from build123d import *

# Parameters (mm, degrees)
BOSS_EXTRUDE1_DEPTH = 19
SKETCH2_R           = 1.905
CUT_EXTRUDE1_DEPTH  = 10.16
CHAMFER1_SIZE       = 1.016
CHAMFER2_SIZE       = 0.254
CHAMFER3_SIZE       = 1.016


with BuildPart() as part:
    # Sketch1 → Boss-Extrude1 (new body)
    with BuildSketch(Plane(origin=(0, 0, 0), x_dir=(0, 0, -1), z_dir=(1, 0, 0))):
        with BuildLine():
            Line((6.25, -13.87), (-25.5, -13.87))
            Line((-25.5, -13.87), (-25.5, 38))
            Line((-25.5, 38), (25.5, 38))
            Line((25.5, 38), (25.5, 24.08))
            Line((25.5, 24.08), (-6.25, 24.08))
            ThreePointArc((-6.25, 24.08), (-11.33, 19), (-6.25, 13.92))
            Line((-6.25, 13.92), (25.5, 13.92))
            Line((25.5, 13.92), (25.5, -38))
            Line((25.5, -38), (-25.5, -38))
            Line((-25.5, -38), (-25.5, -24.03))
            Line((-25.5, -24.03), (6.25, -24.03))
            ThreePointArc((6.25, -24.03), (11.33, -18.95), (6.25, -13.87))
        make_face()
    extrude(amount=BOSS_EXTRUDE1_DEPTH)

    # Sketch2 → Cut-Extrude1 (cut)
    with BuildSketch(Plane.XZ.offset(38)):
        with Locations(Location((9.5, 12, 0), (0, 0, 270))):
            Circle(SKETCH2_R)
        with Locations(Location((9.5, -12, 0), (0, 0, 90))):
            Circle(SKETCH2_R)
    cut_extrude1 = extrude(amount=-CUT_EXTRUDE1_DEPTH, mode=Mode.SUBTRACT)

    # Chamfer1
    chamfer1_edges = [part.edges().sort_by_distance(p)[0] for p in [
        (9.5, -38, 13.905),
        (9.5, -38, -13.905),
    ]]
    chamfer(chamfer1_edges, length=CHAMFER1_SIZE)

    # Chamfer2
    chamfer2_edges = [part.edges().sort_by_distance(p)[0] for p in [
        (19, -18.95, -11.33),
        (0, 12.065, 25.5),
        (0, 38, 0),
        (0, 31.04, -25.5),
        (0, 24.08, -9.625),
        (19, -24.03, 9.625),
        (0, 19, 11.33),
        (0, 13.92, -9.625),
        (0, -12.04, -25.5),
        (0, -38, 0),
        (0, -31.015, 25.5),
        (0, -24.03, 9.625),
        (0, -18.95, -11.33),
        (0, -13.87, 9.625),
        (19, -31.015, 25.5),
        (9.5, -13.87, 25.5),
        (9.5, 38, 25.5),
        (9.5, 38, -25.5),
        (9.5, 24.08, -25.5),
        (9.5, 13.92, -25.5),
        (9.5, -38, -25.5),
        (9.5, -38, 25.5),
        (9.5, -24.03, 25.5),
        (19, -38, 0),
        (19, -12.04, -25.5),
        (19, 13.92, -9.625),
        (19, 19, 11.33),
        (19, 24.08, -9.625),
        (19, 31.04, -25.5),
        (19, 38, 0),
        (19, -13.87, 9.625),
        (19, 12.065, 25.5),
    ]]
    chamfer(chamfer2_edges, length=CHAMFER2_SIZE)

    # Mirror3: Cut-Extrude1 across plane
    add(cut_extrude1.mirror(Plane.ZX), mode=Mode.SUBTRACT)

    # Chamfer3
    chamfer3_edges = [part.edges().sort_by_distance(p)[0] for p in [
        (9.5, 38, 13.905),
        (9.5, 38, -13.905),
    ]]
    chamfer(chamfer3_edges, length=CHAMFER3_SIZE)


solid = part.part
Geometry check sheet. Reference: the model listing, model coordinates, mm. A direction names the side the tool comes from. Round coordinates to 2 decimals unless told otherwise and drop trailing zeros. Loops run counter-clockwise (first coordinate to the right, second up) from the corner with the lowest first, then second, coordinate; pieces in that order, holes last. Notation, with made-up numbers: (16.25, -14.75) - (26.25, -14.75) arc R10 ccw to (26.25, 4.25) - close; hole circle Ø5 at (81, -1.5). An arc over 180 degrees is marked (long way). Answer as CSV lines item,"result".
(1) Depth check by flat-ended pin: pin 1 Ø1.9 at (x, z) = (9.5, 12.5) entering from -Y; pin 2 Ø3 at (x, z) = (9.5, 12) entering from +Y; pin 3 Ø4.5 at (x, z) = (9.5, -12) entering from -Y; pin 4 Ø8 at (y, z) = (18, -16) entering from +X. Enter the tip coordinate at first touch or a pass-through.
Output values:
pin 1,"stops at y = -27.84"
pin 2,"stops at y = 27.84"
pin 3,"stops at y = -37.33"
pin 4,"passes through"
(2) Set-up check for faces 1 (the face through (9, 24.08, -10)), 2 (the face through (8.928, -32.476, -10.183)), 3 (the face through (9, -13.87, 9)): record each of +Z, -Z, +X, -X, +Y, -Y from which the full face is reachable in a straight line by a thin tool's end or side.
Output values:
face 1,"-Z, +X, -X"
face 2,"-Y"
face 3,"+Z, +X, -X"
(3) Cross-section at C-C, the plane x = 13.5. Enter the section's corners in (y, z).
Output values:
outline,"(-38, -25.25) - (-37.75, -25.5) - (13.67, -25.5) - (13.92, -25.25) - (13.92, 6.25) arc R5.08 cw to (24.08, 6.25) - (24.08, -25.25) - (24.33, -25.5) - (37.75, -25.5) - (38, -25.25) - (38, 25.25) - (37.75, 25.5) - (-13.62, 25.5) - (-13.87, 25.25) - (-13.87, -6.25) arc R5.08 cw to (-24.03, -6.25) - (-24.03, 25.25) - (-24.28, 25.5) - (-37.75, 25.5) - (-38, 25.25) - close"
(4) Cross-section at B-B, the plane y = 19. Enter the section's corners in (x, z), and give its area (3 significant figures).
Output values:
outline,"(0, 11.58) - (0.25, 11.33) - (18.75, 11.33) - (19, 11.58) - (19, 25.25) - (18.75, 25.5) - (0.25, 25.5) - (0, 25.25) - close"
area,"269 mm²"
(5) Cross-section at A-A, the plane z = -2. Enter the section's corners in (x, y).
Output values:
outline,"(0, -37.75) - (0.25, -38) - (18.75, -38) - (19, -37.75) - (19, -24.28) - (18.75, -24.03) - (0.25, -24.03) - (0, -24.28) - close; (0, -13.62) - (0.25, -13.87) - (18.75, -13.87) - (19, -13.62) - (19, 13.67) - (18.75, 13.92) - (0.25, 13.92) - (0, 13.67) - close; (0, 24.33) - (0.25, 24.08) - (18.75, 24.08) - (19, 24.33) - (19, 37.75) - (18.75, 38) - (0.25, 38) - (0, 37.75) - close"
(6) Release check for a two-part mould opening along X. For faces 4 (the face through (10.072, 32.476, 10.183)), 5 (the face through (0, 1, 0)), 6 (the face through (18.871, -19.064, -11.454)), 7 (the face through (9, -31, 25.5)) record: released by +X, released by -X, zero draft, split by the parting line, or undercut.
Output values:
face 4,"undercut"
face 5,"released by -X"
face 6,"released by +X"
face 7,"zero draft"
(7) Material ranges on line 1 along Y through (x, z) = (8.5, 2.5); line 2 along Y through (x, z) = (3.5, 23); line 3 along Y through (x, z) = (13.75, -22), recorded low to high.
Output values:
line 1,"y = -38 to -24.03, -13.87 to 13.92, 24.08 to 38"
line 2,"y = -38 to -24.03, -13.87 to 38"
line 3,"y = -38 to 13.92, 24.08 to 38"
